Input: part model. Units: mm. Frame: model coordinates. Coordinates: 2 decimals unless noted, no trailing zeros. Loops run counter-clockwise (first coordinate to the right, second up) from the corner with the lowest first, then second, coordinate; pieces in that order, holes last. Notation, with made-up numbers: (19, 84.25) - (24, 84.25) arc R14 cw to (24, 97.25) - close; hole circle Ø11 at (8.25, -34). An arc over 180 degrees is marked (long way). Write item = value, one per line. Start each with the question number.
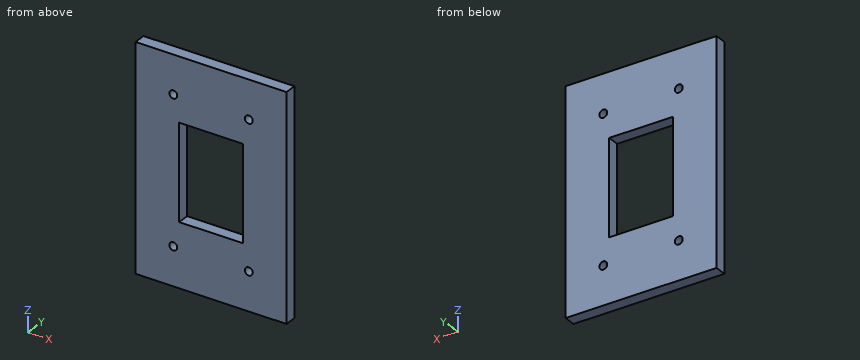
from build123d import *

# Parameters (mm, degrees)
SKETCH1_W               = 241.3
SKETCH1_H               = 355.6
BOSS_EXTRUDE1_DEPTH     = 9.525
SKETCH2_R               = 6.35
CUT_EXTRUDE1_DEPTH      = 20.05
SKETCH3_W               = 101.6
SKETCH3_H               = 152.4
CUT_EXTRUDE2_DEPTH      = 1
CUT_EXTRUDE2_DEPTH_BACK = 20.05


with BuildPart() as part:
    # Sketch1 → Boss-Extrude1 (new body, symmetric)
    with BuildSketch(Plane(origin=(0, 0, 0), x_dir=(1, 0, 0), z_dir=(0, 1, 0))):
        Rectangle(SKETCH1_W, SKETCH1_H)
    extrude(amount=BOSS_EXTRUDE1_DEPTH, both=True)

    # Sketch2 → Cut-Extrude1 (cut, through all)
    with BuildSketch(Plane(origin=(0, 9.525, 0), x_dir=(1, 0, 0), z_dir=(0, 1, 0))):
        with Locations((-60.325, 116.459)):
            Circle(SKETCH2_R)
        with Locations((60.325, 116.459)):
            Circle(SKETCH2_R)
        with Locations((60.325, -116.459)):
            Circle(SKETCH2_R)
        with Locations((-60.325, -116.459)):
            Circle(SKETCH2_R)
    extrude(amount=-CUT_EXTRUDE1_DEPTH, mode=Mode.SUBTRACT)

    # Sketch3 → Cut-Extrude2 (cut, two sides)
    with BuildSketch(Plane(origin=(0, 9.525, 0), x_dir=(1, 0, 0), z_dir=(0, 1, 0))) as cut_extrude2_sk:
        Rectangle(SKETCH3_W, SKETCH3_H)
    extrude(amount=CUT_EXTRUDE2_DEPTH, mode=Mode.SUBTRACT)
    extrude(cut_extrude2_sk.sketch, amount=-CUT_EXTRUDE2_DEPTH_BACK, mode=Mode.SUBTRACT)


solid = part.part
Item 1: Ray query, line 1 (Z direction, x = 27.5, y = -3.75); line 2 (X direction, y = 4.75, z = -18); line 3 (X direction, y = -6.5, z = -114.5). Return the intervals inside material, ascending.
Item 2: Cut plane C-C on y = 1.75. Return loops of the section in (x, z) (3 decimals), plus the area to 3 significant figures.
Item 3: Cut plane A-A on x = 32.5. Return loops of the section in (y, z) (3 decimals), plus the area to 3 significant figures.
Item 4: Cut plane B-B on z = 25. Return loops of the section in (x, y) (3 decimals), plus the area to 3 significant figures.
Recorded:
q1.line_1 = -177.8 to -76.2, 76.2 to 177.8
q1.line_2 = -120.65 to -50.8, 50.8 to 120.65
q1.line_3 = -120.65 to -66.37, -54.28 to 54.28, 66.37 to 120.65
q2.outline = (-120.65, -177.8) - (120.65, -177.8) - (120.65, 177.8) - (-120.65, 177.8) - close; hole circle Ø12.7 at (-60.325, -116.459); hole circle Ø12.7 at (-60.325, 116.459); hole (-50.8, -76.2) - (50.8, -76.2) - (50.8, 76.2) - (-50.8, 76.2) - close; hole circle Ø12.7 at (60.325, -116.459); hole circle Ø12.7 at (60.325, 116.459)
q2.area = 69,800 mm²
q3.outline = (-9.525, -177.8) - (9.525, -177.8) - (9.525, -76.2) - (-9.525, -76.2) - close; (-9.525, 76.2) - (9.525, 76.2) - (9.525, 177.8) - (-9.525, 177.8) - close
q3.area = 3,870 mm²
q4.outline = (-120.65, -9.525) - (-50.8, -9.525) - (-50.8, 9.525) - (-120.65, 9.525) - close; (50.8, -9.525) - (120.65, -9.525) - (120.65, 9.525) - (50.8, 9.525) - close
q4.area = 2,660 mm²
